```python
from build123d import *

# Parameters (mm, degrees)
CHAMFER1_SIZE         = 0.5
CHAMFER2_SIZE         = 0.3
CHAMFER2_SIZE2        = 0.173205081
CHAMFER2_PART_2_SIZE  = 0.3
CHAMFER2_PART_2_SIZE2 = 0.173205081
CHAMFER2_PART_3_SIZE  = 0.3
CHAMFER2_PART_3_SIZE2 = 0.173205081
CHAMFER2_PART_4_SIZE  = 0.3
CHAMFER2_PART_4_SIZE2 = 0.173205081
SKETCH2_W             = 23.197150539
SKETCH2_H             = 11.802059046
CUT_EXTRUDE1_DEPTH    = 50
CHAMFER3_SIZE         = 0.5


with BuildPart() as part:
    # Sketch1 → Revolve1 (revolve)
    with BuildSketch(Plane(origin=(0, 0, 0), x_dir=(1, 0, 0), z_dir=(0, 1, 0))):
        Polygon((-1, 0), (-4, 0), (-4, -121), (-1, -121), (-1, -119), (0, -119), (0, -2), (-1, -2), align=None)
    revolve(axis=Axis((0, 0, 119), (0, 0, -1)))

    # Chamfer1
    chamfer1_edges = [part.edges().sort_by_distance(p)[0] for p in [
        (4, 0, 121),
        (4, 0, 0),
    ]]
    chamfer(chamfer1_edges, length=CHAMFER1_SIZE)

    # Chamfer2
    chamfer2_edges = [part.edges().sort_by_distance(p)[0] for p in [
        (1, 0, 2),
    ]]
    chamfer2_side = [part.faces().sort_by_distance(p)[0] for p in [
        (0, 0, 2),
    ]]
    chamfer(chamfer2_edges, length=CHAMFER2_SIZE, length2=CHAMFER2_SIZE2, reference=chamfer2_side[0])

    # Chamfer2 part 2
    chamfer2_part_2_edges = [part.edges().sort_by_distance(p)[0] for p in [
        (1, 0, 119),
    ]]
    chamfer2_part_2_side = [part.faces().sort_by_distance(p)[0] for p in [
        (1, 0, 120),
    ]]
    chamfer(chamfer2_part_2_edges, length=CHAMFER2_PART_2_SIZE, length2=CHAMFER2_PART_2_SIZE2, reference=chamfer2_part_2_side[0])

    # Chamfer2 part 3
    chamfer2_part_3_edges = [part.edges().sort_by_distance(p)[0] for p in [
        (1, 0, 121),
    ]]
    chamfer2_part_3_side = [part.faces().sort_by_distance(p)[0] for p in [
        (3.401005051, 0, 121),
    ]]
    chamfer(chamfer2_part_3_edges, length=CHAMFER2_PART_3_SIZE, length2=CHAMFER2_PART_3_SIZE2, reference=chamfer2_part_3_side[0])

    # Chamfer2 part 4
    chamfer2_part_4_edges = [part.edges().sort_by_distance(p)[0] for p in [
        (1, 0, 0),
    ]]
    chamfer2_part_4_side = [part.faces().sort_by_distance(p)[0] for p in [
        (1, 0, 1),
    ]]
    chamfer(chamfer2_part_4_edges, length=CHAMFER2_PART_4_SIZE, length2=CHAMFER2_PART_4_SIZE2, reference=chamfer2_part_4_side[0])

    # Sketch2 → Cut-Extrude1 (cut)
    with BuildSketch(Plane(origin=(0, 28.2, 0), x_dir=(1, 0, 0), z_dir=(0, 1, 0))):
        with Locations((2.541571207, -122.251029523)):
            Rectangle(SKETCH2_W, SKETCH2_H)
    extrude(amount=-CUT_EXTRUDE1_DEPTH, mode=Mode.SUBTRACT)

    # Chamfer3
    chamfer3_edges = [part.edges().sort_by_distance(p)[0] for p in [
        (4, 0, 116.35),
    ]]
    chamfer(chamfer3_edges, length=CHAMFER3_SIZE)


solid = part.part
```
The listing builds one solid part. Answer for the finished solid, in the listing's coordinates (mm). Round coordinates to 2 decimals unless told otherwise and drop trailing zeros. Loops run counter-clockwise (first coordinate to the right, second up) from the corner with the lowest first, then second, coordinate; pieces in that order, holes last. Notation, with made-up numbers: (78.5, 89.25) - (133.5, 89.25) arc R11 cw to (133.5, 101.25) - close; hole circle Ø3 at (-24.75, -17.5). An arc over 180 degrees is marked (long way). Return JSON: item names as keys, results as strings. Group by question number.
1. Each of these flat-tipped pins is pushed along its axis until it touches: P1, Ø1.5, axis at y = 1, z = 30.5, coming from the -X side; P2, Ø1, axis at x = -3, z = 94.5, coming from the +Y side; P3, Ø2, axis at x = -3, z = 93, coming from the +Y side. Where does it stop, or does it pass through?
2. The mould has two halves that part along Y. Classify faces 1 (the cylindrical face through (0, -1, 1)), 2 (the cylindrical face through (0.867, -3.905, 58.982)), 3 (the flat face through (0, -2, 0)): pulls with the +Y half, pulls with the -Y half, needs draft (parallel to the pull), parting line crosses it, or undercut.
3. Consider probe 1 along Z at (x, y) = (-0.5, 0.5); probe 2 along Y at (x, z) = (0.25, 87.5); probe 3 along Z at (x, y) = (3.5, 0.25). Determine where each line is inside the solid, lowest interval first.
4. The part is cut by section A-A on z = 95.5. Determine the outline of the cut face in (x, y), then the cut area to 3 significant figures.
Resolved:
{
 "1": {"P1": "stops at x = -3.99", "P2": "stops at y = 3.12", "P3": "stops at y = 3.46"},
 "2": {"face 1": "undercut", "face 2": "parting line crosses it", "face 3": "needs draft"},
 "3": {"probe 1": "z = 2 to 116.35", "probe 2": "y = -3.99 to 3.99", "probe 3": "z = 0.01 to 116.34"},
 "4": {"outline": "circle Ø8 at (0, 0)", "area": "50.3 mm²"}
}
